from build123d import *

# Parameters (mm, degrees)
SKETCH1_W           = 55
SKETCH1_H           = 45
BOSS_EXTRUDE1_DEPTH = 3
SKETCH2_W           = 10
SKETCH2_H           = 13
BOSS_EXTRUDE2_DEPTH = 12.5
SKETCH3_R           = 1.75
CUT_EXTRUDE1_DEPTH  = 13.5
FILLET1_R           = 6
CHAMFER1_SIZE       = 12
FILLET3_R           = 1
SKETCH4_W           = 20
SKETCH4_H           = 5
CUT_EXTRUDE3_DEPTH  = 5
SKETCH7_R           = 1.75
CUT_EXTRUDE4_DEPTH  = 5
BOSS_EXTRUDE4_DEPTH = 3


with BuildPart() as part:
    # Sketch1 → Boss-Extrude1 (new body)
    with BuildSketch(Plane.XY):
        with Locations((-16.936997319, -3.156836461)):
            Rectangle(SKETCH1_W, SKETCH1_H)
    extrude(amount=BOSS_EXTRUDE1_DEPTH)

    # Sketch2 → Boss-Extrude2 (add)
    with BuildSketch(Plane(origin=(0, 0, 0), x_dir=(-1, 0, 0), z_dir=(0, 0, -1))):
        with Locations((-5.563002681, -3.156836461)):
            Rectangle(SKETCH2_W, SKETCH2_H)
    extrude(amount=BOSS_EXTRUDE2_DEPTH)

    # Sketch3 → Cut-Extrude1 (cut)
    with BuildSketch(Plane(origin=(0, 3.343163539, 0), x_dir=(1, 0, 0), z_dir=(0, 1, 0))):
        with Locations(Location((5.563002681, 7.5, 0), (0, 0, 180))):
            Circle(SKETCH3_R)
    extrude(amount=-CUT_EXTRUDE1_DEPTH, mode=Mode.SUBTRACT)

    # Fillet1
    fillet1_edges = [part.edges().sort_by_distance(p)[0] for p in [
        (10.563002681, -3.156836461, -12.5),
    ]]
    fillet(fillet1_edges, radius=FILLET1_R)

    # Chamfer1
    chamfer1_edges = [part.edges().sort_by_distance(p)[0] for p in [
        (0.563002681, -3.156836461, 0),
    ]]
    chamfer(chamfer1_edges, length=CHAMFER1_SIZE)

    # Fillet3
    # the kernel refuses this fillet: 1 mm, written as the material it takes off along each edge
    with BuildSketch(Plane(origin=(0.563002681, 5.508227048, -12.5), x_dir=(1, 0, 0), z_dir=(0, -1, 0))) as fillet3_piece_1:
        with BuildLine():
            CenterArc((0.866025404, 1), FILLET3_R, 210, 60)
            Line((0, 0.5), (-0.017320508, 0.49))
            ThreePointArc((-0.017320508, 0.49), (-0.02, 0.25), (-0.02, 0))
            Line((-0.02, 0), (0, -0.02))
            Line((0, -0.02), (0.866025404, -0.02))
            Line((0.866025404, -0.02), (0.866025404, 0))
        make_face()
    extrude(amount=17.330127019, mode=Mode.SUBTRACT)

    # Sketch4 → Cut-Extrude3 (cut)
    with BuildSketch(Plane(origin=(0, 0, 0), x_dir=(-1, 0, 0), z_dir=(0, 0, -1))):
        with Locations((-5.563002681, 10.343163539)):
            Rectangle(SKETCH4_W, SKETCH4_H)
    cut_extrude3 = extrude(amount=-CUT_EXTRUDE3_DEPTH, mode=Mode.SUBTRACT)

    # Mirror2: Cut-Extrude3 across plane
    add(cut_extrude3.mirror(Plane.ZX.offset(-3.156836461)), mode=Mode.SUBTRACT)

    # Sketch7 → Cut-Extrude4 (cut)
    with BuildSketch(Plane(origin=(0, 0, 0), x_dir=(-1, 0, 0), z_dir=(0, 0, -1))):
        with Locations((-5.563002681, 16.343163539)):
            Circle(SKETCH7_R)
        with Locations((39.436997319, 16.343163539)):
            Circle(SKETCH7_R)
        with Locations(Location((39.436997319, -22.656836461, 0), (0, 0, 180))):
            Circle(SKETCH7_R)
        with Locations(Location((-5.563002681, -22.656836461, 0), (0, 0, 180))):
            Circle(SKETCH7_R)
    extrude(amount=-CUT_EXTRUDE4_DEPTH, mode=Mode.SUBTRACT)

    # Sketch8 → Boss-Extrude4 (add)
    with BuildSketch(Plane(origin=(0, 0, 0), x_dir=(-1, 0, 0), z_dir=(0, 0, -1))):
        Polygon((44.436997319, 6.843163539), (51.936997319, 6.843163539), (51.936997319, 9.343163539), (59.436997319, 4.091607002), (59.436997319, -10.405279925), (51.936997319, -15.656836461), (51.936997319, -13.156836461), (44.436997319, -13.156836461), align=None)
    extrude(amount=-BOSS_EXTRUDE4_DEPTH)


solid = part.part
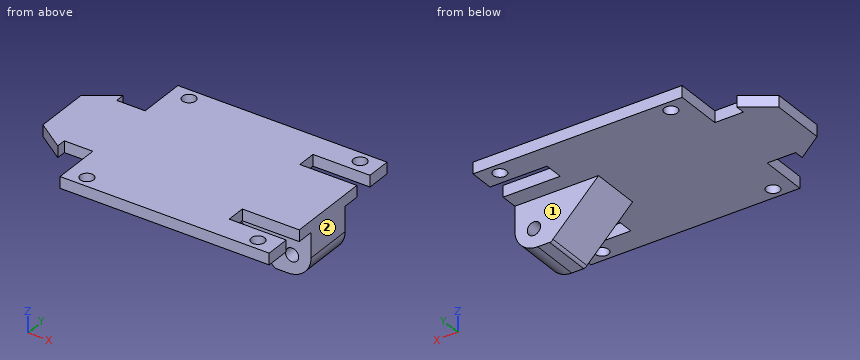
Part model, mm, in its own coordinate system. Face numbers are marked on the shaded views. A direction names the side the tool comes from. Round coordinates to 2 decimals unless told otherwise and drop trailing zeros. Write each loop counter-clockwise with the first axis right and the second up, starting at its lowest first coordinate (ties: lowest second). Pieces come first, ordered by that corner, then holes. Notation, with made-up numbers: (4.5, 70.5) - (38.5, 70.5) arc R29 cw to (38.5, 101.5) - close; hole circle Ø8 at (40, -31). An arc over 180 degrees is marked (long way). Use CSV: the item, a comma, the result in double quotes.
Item 1: Wall check: L1, parallel to X at y = -23, z = 0.75; L2, parallel to X at y = 11, z = 0.5; L3, parallel to Z at x = -37, y = 9. Give the ranges that are in metal, low to high.
Results list:
L1,"x = -44.44 to -41.15, -37.72 to 3.85, 7.28 to 10.56"
L2,"x = -44.44 to -4.44"
L3,"z = 0 to 3"
Item 2: Tool access for the marked faces 1 and 2: list every direction of +Z, -Z, +X, -X, +Y, -Y with a clear straight run to the whole face (end or side of a thin tool).
Results list:
face 1,"-Z, +X, -X, +Y"
face 2,"+Z, -Z, +X, +Y, -Y"
Item 3: Slice it at B-B, the plane x = -1.5. Write the cut outline in (y, z), then the cut area to 3 significant figures.
Results list:
outline,"(-25.66, 0) - (-19.16, 0) - (-19.16, 3) - (-25.66, 3) - close; (-14.16, 0) - (-9.66, 0) - (-9.66, -9.94) - (3.34, -9.94) - (3.34, 0) - (7.84, 0) - (7.84, 3) - (-14.16, 3) - close; (12.84, 0) - (19.34, 0) - (19.34, 3) - (12.84, 3) - close"
area,"234 mm²"
Item 4: Slice it at A-A, the plane y = -8. Write the cut outline in (x, z), then the cut area to 3 significant figures.
Results list:
outline,"(-59.44, 0) - (-11.44, 0) - (0.56, -12) arc R1 ccw to (1.43, -12.5) - (4.56, -12.5) arc R6 ccw to (10.56, -6.5) - (10.56, 3) - (-59.44, 3) - close; hole circle Ø3.5 at (5.56, -7.5)"
area,"390 mm²"
Item 5: Slice it at C-C, the plane z = -7.5. Write the cut outline in (x, y).
Results list:
outline,"(-3.94, -9.66) - (3.81, -9.66) - (3.81, 3.34) - (-3.94, 3.34) - close; (7.31, -9.66) - (10.48, -9.66) - (10.48, 3.34) - (7.31, 3.34) - close"
Item 6: Slice it at D-D, the plane x = -22. Write the cut outline in (y, z), then the cut area to 3 significant figures.
Results list:
outline,"(-25.66, 0) - (19.34, 0) - (19.34, 3) - (-25.66, 3) - close"
area,"135 mm²"
Item 7: Flat gauge pins, fed straight in: P1, Ø4, axis at y = -5.5, z = -10.5, coming from the -X side; P2, Ø3.5, axis at y = -16.5, z = 1, coming from the +X side; P3, Ø4, axis at x = 0, z = -3.5, coming from the +Y side. Where does each tip first touch, or does it go through?
Results list:
P1,"stops at x = -2.94"
P2,"stops at x = -4.44"
P3,"stops at y = 3.34"
